Job drawing, mm, ordinate dimensions from the low corner. One solid piece. Give positions to 0.01 mm unless a question says otherwise; leave off trailing zeros. Write each loop counter-clockwise with the first axis right and the second up, starting at its lowest first coordinate (ties: lowest second). Pieces come first, ordered by that corner, then holes. Notation, with made-up numbers: M -37.75,-26.75 L 12.25,-26.75 A15 ccw 12.25,-22.75 Z; hole C 52.25,29 d8. An arc over 180 degrees is marked long. Answer as CSV lines item,"result". Start each with the question number.
Item 1: Pin check, flat tips, straight feed: pin 1 (1.5 mm diameter, centred on x = 6.5, z = 30.5, fed in from +Y); pin 2 (12 mm diameter, centred on x = 14, z = 16, fed in from +Y); pin 3 (10 mm diameter, centred on y = 13.5, z = 16, fed in from -X). Stop position of each tip, or through.
Item 2: Wall check: L1, parallel to X at y = 3.5, z = 35 (1 decimal); L2, parallel to Y at x = 16.75, z = 4; L3, parallel to Y at x = 2, z = 38 (1 decimal). Give the ranges that are in metal, low to high. Write a range as from..to.
Item 3: Two-plate mould, pull along Z, no slides. Class the marked faces 1, 2 and 3: +Z half, -Z half, draft (parallel to the pull), parting line (faces both ways), or undercut.
Item 4: Band-saw the part on D-D, the plane z = 37.5. List the corners of the cut face in (x, y) (1 decimal).
Item 5: Band-saw the part on C-C, the plane z = 25.5. List the corners of the cut face in (x, y).
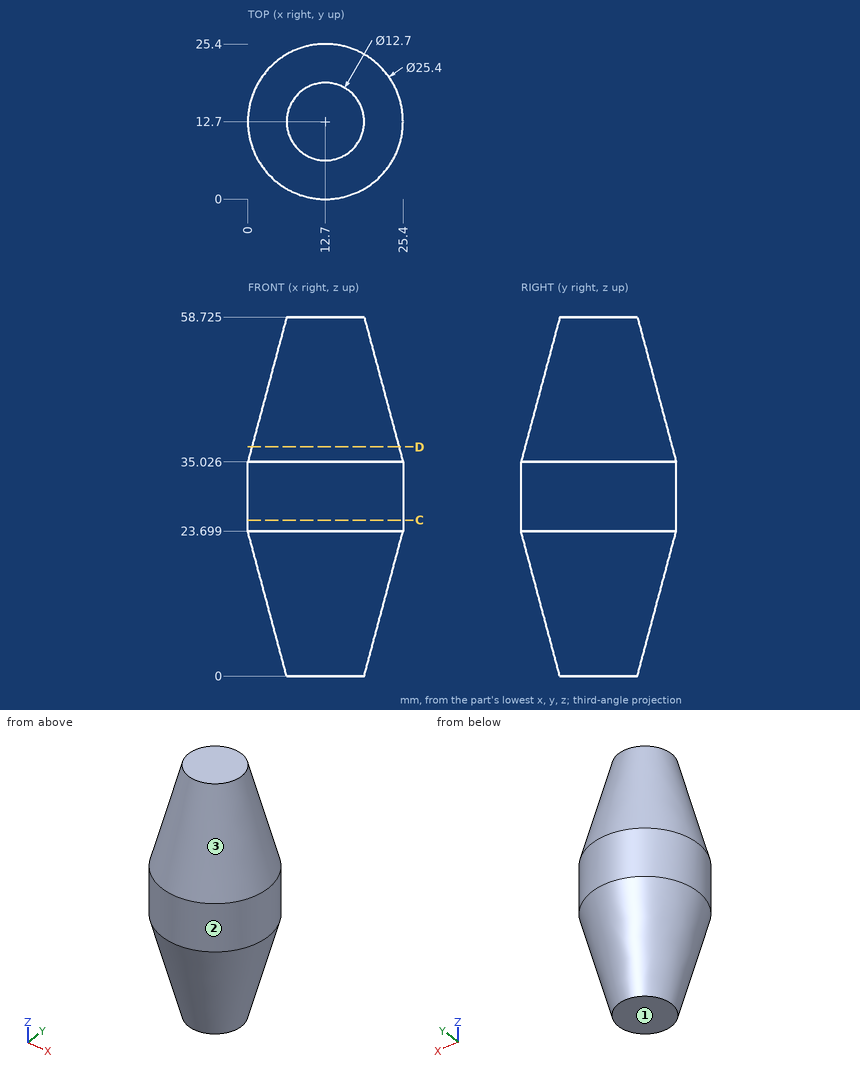
Output:
1,pin 1,"y = 24.17"
1,pin 2,"y = 24.92"
1,pin 3,"x = 0.73"
2,L1,"3.9..21.5"
2,L2,"6.48..18.92"
2,L3,"7.5..17.9"
3,face 1,"-Z half"
3,face 2,"draft"
3,face 3,"+Z half"
4,outline,"C 12.7,12.7 d24.1"
5,outline,"C 12.7,12.7 d25.4"
